Autodesk Inventor part; units mm, degrees
ref_plane "YZ Plane" through (0, 0, 0) normal (1, 0, 0) x (0, 1, 0)
ref_plane "XZ Plane" through (0, 0, 0) normal (0, 1, 0) x (-1, 0, 0)
ref_plane "XY Plane" through (0, 0, 0) normal (0, 0, 1) x (1, 0, 0)
sketch "スケッチ1" plane through (0, 0, 0) normal (0, 0, 1) x (1, 0, 0)
  line L0 (0, 11) -> (-4, 11)
  line L1 (-4, 11) -> (-4, 9.5)
  line L2 (-4, 9.5) -> (-2, 9.5)
  line L3 (-2, 9.5) -> (-2, 0)
  line L4 (-2, 0) -> (0, 0)
  line L5 (0, 0) -> (0, 11)
  line L6 (0, -2.2) -> (0, 13.2)
  dimension "d0" = 4
  dimension "d1" = 1.5
  dimension "d2" = 2
  dimension "d3" = 11
revolve "回転1" add sketch "スケッチ1" angle 360 about axis through (0, -10, 0) along (0, 1, 0)
mirror "ミラー1" about plane through (-2, 0, 0) normal (0, -1, 0) of "回転1"
ref_plane "作業平面1" through (0, 0, 0) normal (0, -1, 0) x (1, 0, 0)
properties part number "castshaft" material "アルミニウム 6061"
Input: part model. Units: mm. Frame: model coordinates. A direction names the side the tool comes from. Coordinates: 2 decimals unless noted, no trailing zeros. Write each loop counter-clockwise with the first axis right and the second up, starting at its lowest first coordinate (ties: lowest second). Pieces come first, ordered by that corner, then holes. Notation, with made-up numbers: (-18.5, 86.25) -> (28.5, 86.25) arc R17 cw to (28.5, 93.25) -> close; hole circle Ø3 at (-16.5, 36.25). An arc over 180 degrees is marked (long way). Answer as a JSON object with one key per item and string values.
1. Section A-A on z = 0. Return the cut outline in (x, y), then the cut area to 3 significant figures.
Result set:
{"outline": "(-4, -11) -> (4, -11) -> (4, -9.5) -> (2, -9.5) -> (2, 9.5) -> (4, 9.5) -> (4, 11) -> (-4, 11) -> (-4, 9.5) -> (-2, 9.5) -> (-2, -9.5) -> (-4, -9.5) -> close", "area": "100 mm2"}
2. Section D-D on z = 3.25. Return the cut outline in (x, y).
Result set:
{"outline": "(-2.33, -11) -> (2.33, -11) -> (2.33, -9.5) -> (-2.33, -9.5) -> close; (-2.33, 9.5) -> (2.33, 9.5) -> (2.33, 11) -> (-2.33, 11) -> close"}
3. Mould query, pull axis Y, two halves, no side actions, for faces 3 (the face through (2, 9.5, -1)), 4 (the face through (0.867, 10.24, 3.905)), 5 (the face through (0, -11, 0)). Classes: released by +Y, released by -Y, zero draft, split by the parting line, or undercut.
Result set:
{"face 3": "undercut", "face 4": "zero draft", "face 5": "released by -Y"}
4. Section B-B on x = 3. Return the cut outline in (y, z), then the cut area to 3 significant figures.
Result set:
{"outline": "(-11, -2.65) -> (-9.5, -2.65) -> (-9.5, 2.65) -> (-11, 2.65) -> close; (9.5, -2.65) -> (11, -2.65) -> (11, 2.65) -> (9.5, 2.65) -> close", "area": "15.9 mm2"}
5. Access query for faces 1 (the face through (0.867, -10.24, -3.905)), 2 (the face through (-2, -9.5, -1)). Directions: +Z, -Z, +X, -X, +Y, -Y. A direction counts if a zero-diameter tool reaches every point of the face in a straight line with its end or side. Return the directions, or none.
Result set:
{"face 1": "+Y, -Y", "face 2": "none"}
6. Section C-C on y = 5.25. Return the cut outline in (x, z).
Result set:
{"outline": "circle Ø4 at (0, 0)"}
7. First-contact query: P1, Ø1, axis at y = 4, z = 3, coming from the +X side; P2, Ø1, axis at x = 0, y = -5, coming from the -Z side. Flat tips, straight axial feed; report the tip coordinate or a pass-through.
Result set:
{"P1": "passes through", "P2": "stops at z = -2"}
8. Material intervals for line 1 (Y direction, x = 1.25, z = 2.25); line 2 (Z direction, x = -1, y = 3.25); line 3 (X direction, y = -4.75, z = -1.75), sorted ascending. Write a range as from..to.
Result set:
{"line 1": "y = -11..-9.5, 9.5..11", "line 2": "z = -1.73..1.73", "line 3": "x = -0.97..0.97"}
